Can you work these out from the drawing? Everything is in mm from the part's minimum corner. Give positions to 0.01 mm unless a question says otherwise; leave off trailing zeros. Write each loop counter-clockwise with the first axis right and the second up, starting at its lowest first coordinate (ties: lowest second). Pieces come first, ordered by that corner, then holes. Notation, with made-up numbers: (59.25, 75.25) - (92.25, 75.25) arc R23 cw to (92.25, 95.25) - close; hole circle Ø3 at (82, 42). An arc over 180 degrees is marked (long way). Use a Markdown table: item, result.
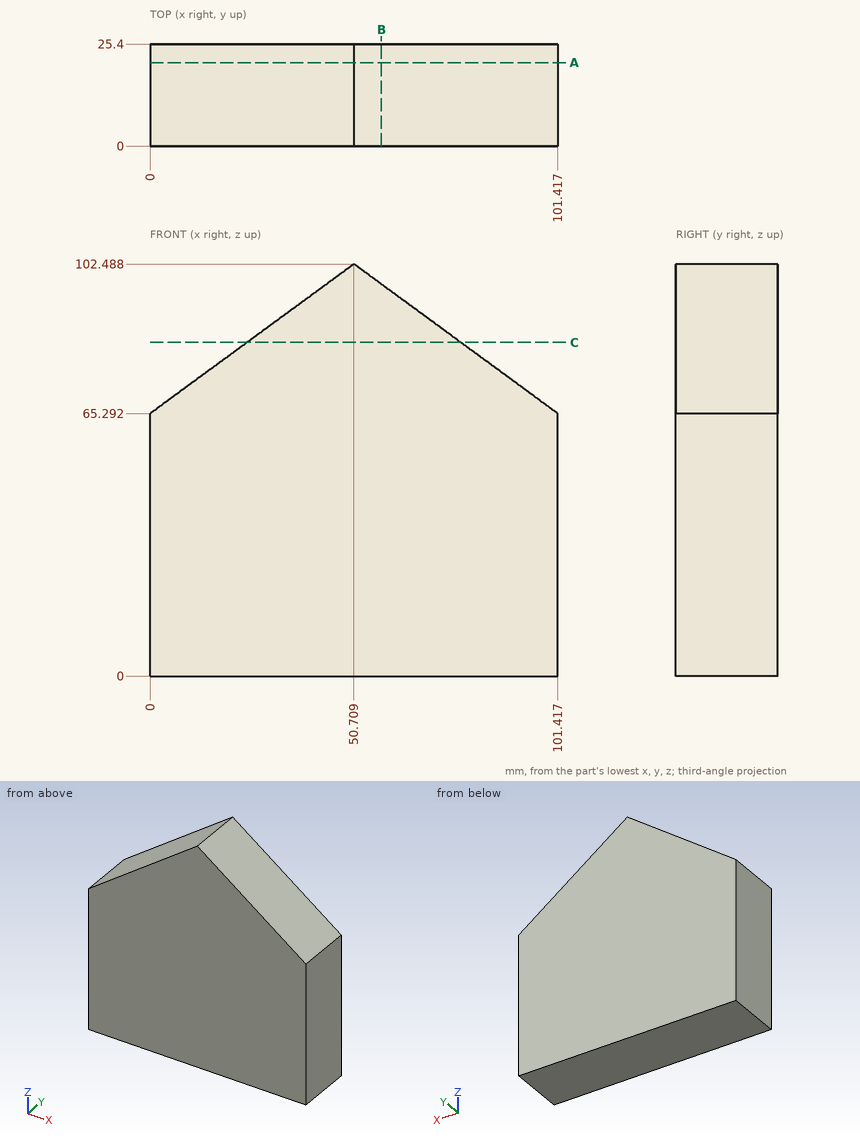
Item 1: If we section it at C-C, the plane z = 83: Write out the boundary of the cut face in (x, y), plus the area to 3 significant figures.
Values:
| item | result |
|---|---|
| outline | (24.14, 0) - (77.28, 0) - (77.28, 25.4) - (24.14, 25.4) - close |
| area | 1,350 mm2 |
Item 2: If we section it at B-B, the plane x = 57.5: Write out the boundary of the cut face in (y, z), plus the area to 3 significant figures.
Values:
| item | result |
|---|---|
| outline | (0, 0) - (25.4, 0) - (25.4, 97.51) - (0, 97.51) - close |
| area | 2,480 mm2 |
Item 3: If we section it at A-A, the plane y = 20.75: Write out the boundary of the cut face in (x, z).
Values:
| item | result |
|---|---|
| outline | (0, 0) - (101.42, 0) - (101.42, 65.29) - (50.71, 102.49) - (0, 65.29) - close |
Item 4: I need wall thicknesses on line 1 along X through (y, z) = (7.25, 98) (1 decimal); line 2 along Z through (x, y) = (84.5, 9.25); line 3 along X through (y, z) = (14.5, 86.5) (1 decimal). Which ranges of each line are inside material? Lowest first, please. Write a range as [from, to].
Values:
| item | result |
|---|---|
| line 1 | x = [44.6, 56.8] |
| line 2 | z = [0, 77.7] |
| line 3 | x = [28.9, 72.5] |
Item 5: Will these pins go through, and if not, where does the flat tip stop? pin 1 Ø12 at (x, z) = (68, 21.5) entering from -Y; pin 2 Ø8 at (y, z) = (16.5, 81.5) entering from -X; pin 3 Ø1 at (y, z) = (18.5, 75.5) entering from -X (1 decimal).
Values:
| item | result |
|---|---|
| pin 1 | stops at y = 0 |
| pin 2 | stops at x = 16.64 |
| pin 3 | stops at x = 13.2 |
